```python
from build123d import *

# Parameters (mm, degrees)
BOSS_EXTRUDE1_DEPTH     = 48
CUT_EXTRUDE1_DEPTH      = 71.615550563
CUT_EXTRUDE1_DEPTH_BACK = 45
SKETCH3_R               = 6
SKETCH3_R_2             = 1.5
CUT_EXTRUDE2_DEPTH      = 71.615550563
SKETCH4_R               = 2
CUT_EXTRUDE3_DEPTH      = 70.146246697


with BuildPart() as part:
    # Sketch1 → Boss-Extrude1 (new body)
    with BuildSketch(Plane(origin=(0, 0, 0), x_dir=(1, 0, 0), z_dir=(0, 1, 0))):
        with BuildLine():
            Line((37.5, 0), (12.5, 0))
            ThreePointArc((12.5, 0), (0, -4.774575141), (-12.5, 0))
            Line((-12.5, 0), (-37.5, 0))
            Line((-37.5, 0), (-37.5, 3))
            Line((-37.5, 3), (-21.75, 3))
            Line((-21.75, 3), (-21.75, 13.975424859))
            ThreePointArc((-21.75, 13.975424859), (0, 35.725424859), (21.75, 13.975424859))
            Line((21.75, 13.975424859), (21.75, 3))
            Line((21.75, 3), (37.5, 3))
            Line((37.5, 3), (37.5, 0))
        make_face()
    extrude(amount=BOSS_EXTRUDE1_DEPTH)

    # Sketch2 → Cut-Extrude1 (cut, two sides: drawn at the far end of the back side and taken through both)
    with BuildSketch(Plane(origin=(0, 48, 0), x_dir=(1, 0, 0), z_dir=(0, 1, 0)).offset(-CUT_EXTRUDE1_DEPTH_BACK)):
        with BuildLine():
            Line((18.75, -143.272179863), (18.75, 0))
            Line((18.75, 0), (18.75, 13.975424859))
            ThreePointArc((18.75, 13.975424859), (0, 32.725424859), (-18.75, 13.975424859))
            Line((-18.75, 13.975424859), (-18.75, 0))
            Line((-18.75, 0), (-18.75, -143.272179863))
            Line((-18.75, -143.272179863), (-18.75, -429.81653959))
            Line((-18.75, -429.81653959), (18.75, -429.81653959))
            Line((18.75, -429.81653959), (18.75, -143.272179863))
        make_face()
    extrude(amount=CUT_EXTRUDE1_DEPTH + CUT_EXTRUDE1_DEPTH_BACK, mode=Mode.SUBTRACT)

    # Sketch3 → Cut-Extrude2 (cut, through all)
    with BuildSketch(Plane.XZ):
        with Locations(Location((0, -20.975424859, 0), (0, 0, 270))):
            Circle(SKETCH3_R)
        with Locations(Location((15.5, -13.975424859, 0), (0, 0, 270))):
            Circle(SKETCH3_R_2)
        with Locations(Location((7.75, -27.398818618, 0), (0, 0, 270))):
            Circle(SKETCH3_R_2)
        with Locations(Location((-7.75, -27.398818618, 0), (0, 0, 270))):
            Circle(SKETCH3_R_2)
        with Locations(Location((-15.5, -13.975424859, 0), (0, 0, 270))):
            Circle(SKETCH3_R_2)
        with Locations(Location((-7.75, -0.552031101, 0), (0, 0, 270))):
            Circle(SKETCH3_R_2)
        with Locations(Location((7.75, -0.552031101, 0), (0, 0, 270))):
            Circle(SKETCH3_R_2)
    extrude(amount=-CUT_EXTRUDE2_DEPTH, mode=Mode.SUBTRACT)

    # Sketch4 → Cut-Extrude3 (cut, through all)
    with BuildSketch(Plane(origin=(0, 0, -3), x_dir=(-1, 0, 0), z_dir=(0, 0, -1))):
        with Locations((-30, 6)):
            Circle(SKETCH4_R)
        with Locations((-30, 24)):
            Circle(SKETCH4_R)
        with Locations((-30, 42)):
            Circle(SKETCH4_R)
        with Locations((30, 6)):
            Circle(SKETCH4_R)
        with Locations((30, 24)):
            Circle(SKETCH4_R)
        with Locations((30, 42)):
            Circle(SKETCH4_R)
    extrude(amount=-CUT_EXTRUDE3_DEPTH, mode=Mode.SUBTRACT)


solid = part.part
```
Check sheet for the modelled part. Datum: model origin and axes. Units: mm. A direction names the side the tool comes from. Round coordinates to 2 decimals unless told otherwise and drop trailing zeros. Loops run counter-clockwise (first coordinate to the right, second up) from the corner with the lowest first, then second, coordinate; pieces in that order, holes last. Notation, with made-up numbers: (29, -1.75) - (56, -1.75) arc R20 ccw to (56, 25.25) - close; hole circle Ø10 at (41, 65.25). An arc over 180 degrees is marked (long way). Write item = value, one per line. Start each with the question number.
Q1. Thickness scan on L1, parallel to Y at x = -30, z = -2; L2, parallel to X at y = 31, z = -7; L3, parallel to X at y = 45.5, z = -2.5. Record the ranges inside material, lowest first.
Q2. Depth check by flat-ended pin: P1, Ø2, axis at x = -12.5, y = 25.5, coming from the -Z side; P2, Ø3.5, axis at x = -7.75, z = -27.4, coming from the +Y side; P3, Ø15.5, axis at y = 23.5, z = -8.5, coming from the -X side; P4, Ø2.5, axis at x = -7.75, z = -0.55, coming from the +Y side. Enter the tip coordinate at first touch or a pass-through.
Q3. Section check A-A (y = 42). Record the boundary of the cut face in (x, z).
Q4. Section check D-D (z = -9.5). Record the boundary of the cut face in (x, y).
Q5. Section check C-C (x = 7.75). Record the boundary of the cut face in (y, z), plus the area to 3 significant figures.
Q6. Access from +Z, -Z, +X, -X, +Y, -Y to the whole of each face (thin tool, end or side, straight path). Record for faces 1 (the face through (27.8, 23.7, -3)), 2 (the face through (-37.5, 24, -1)), 3 (the face through (1, 0, -11)), 4 (the face through (-27.6, 23.7, 0)), 5 (the face through (0, 3, -10)).
Q7. Release check for a two-part mould opening along X. For faces 6 (the face through (-0.48, 23.66, -35.72)), 7 (the face through (-15.434, 1.479, -12.477)), 8 (the face through (-21.75, 24, -8)), 9 (the face through (3, 48, -33)) record: pulls with the +X half, pulls with the -X half, needs draft (parallel to the pull), parting line crosses it, or undercut.
Q8. Section check B-B (x = 0). Record the boundary of the cut face in (y, z).
Derived:
q1.L1 = 0 to 4, 8 to 22, 26 to 40, 44 to 48
q1.L2 = -21.75 to -18.75, 18.75 to 21.75
q1.L3 = -37.5 to -18.75, 18.75 to 37.5
q2.P1 = -32.44
q2.P2 = 3
q2.P3 = -37.5
q2.P4 = through
q3.outline = (-37.5, -3) - (-32, -3) - (-32, 0) - (-37.5, 0) - close; (-28, -3) - (-21.75, -3) - (-21.75, -13.98) arc R21.75 ccw to (21.75, -13.98) - (21.75, -3) - (28, -3) - (28, 0) - (18.75, 0) - (18.75, -13.98) arc R18.75 cw to (-18.75, -13.98) - (-18.75, 0) - (-28, 0) - close; (32, -3) - (37.5, -3) - (37.5, 0) - (32, 0) - close
q4.outline = (-21.75, 0) - (21.75, 0) - (21.75, 48) - (18.75, 48) - (18.75, 3) - (-18.75, 3) - (-18.75, 48) - (-21.75, 48) - close
q5.outline = (0, -34.3) - (48, -34.3) - (48, -31.05) - (3, -31.05) - (3, -28.9) - (0, -28.9) - close; (0, -25.9) - (3, -25.9) - (3, -2.05) - (0, -2.05) - close; (0, 0.95) - (3, 0.95) - (3, 3.1) - (0, 3.1) - close
q5.area = 240 mm^2
q6.face_1 = -Z, +X, +Y, -Y
q6.face_2 = +Z, -Z, -X, +Y, -Y
q6.face_3 = +Z, -Z, +X, -X, -Y
q6.face_4 = +Z, -X, +Y, -Y
q6.face_5 = +Z, +Y
q7.face_6 = parting line crosses it
q7.face_7 = undercut
q7.face_8 = pulls with the -X half
q7.face_9 = needs draft
q8.outline = (0, -35.73) - (48, -35.73) - (48, -32.73) - (3, -32.73) - (3, -26.98) - (0, -26.98) - close; (0, -14.98) - (3, -14.98) - (3, 4.77) - (0, 4.77) - close
